Input: part model. Units: mm. Frame: model coordinates. A direction names the side the tool comes from. Coordinates: 2 decimals unless noted, no trailing zeros. Loops run counter-clockwise (first coordinate to the right, second up) from the corner with the lowest first, then second, coordinate; pieces in that order, holes last. Notation, with made-up numbers: (-28.5, -16.5) - (15.5, -16.5) arc R25 ccw to (15.5, 2.5) - close; hole circle Ø1 at (20.25, -14). An arc over 180 degrees is marked (long way). Use a Markdown table: item, result. Add a question column.
1. Section query C-C on x = 6. Return the cut outline in (y, z), then the cut area to 3 significant figures.
2. Section query A-A on y = 6. Return the cut outline in (x, z), then the cut area to 3 significant figures.
3. Access query for faces 1 (the face through (8.183, 20, 62)), 2 (the face through (15.183, 20, 62)), 3 (the face through (-23, 2, 52.899)), 4 (the face through (12, 20, -14.605)). Directions: +Z, -Z, +X, -X, +Y, -Y. A direction counts if a zero-diameter tool reaches every point of the face in a straight line with its end or side. Return the directions, or none.
4. Section query D-D on x = -46. Return the cut outline in (y, z).
5. Section query B-B on z = 23. State how many separate pieces and enclosed holes the cut face has, then the cut area to 3 significant figures.
6. Draft query along Z for faces 5 (the face through (17, 2, -7.101)), 6 (the face through (9, 12, 65.399)), 7 (the face through (4.383, 2, 23)), 8 (the face through (-47.817, 20, 23)). Return one class per face: released by +Z, released by -Z, zero draft, split by the parting line, or undercut.
7. Ray query, L1, parallel to Y at x = -18, z = 37.5; L2, parallel to X at y = 29, z = 62; L3, parallel to X at y = 30, z = 59. Return the intervals inside material, ascending. Write a range as [from, to].
8. Contact query for flat-ended pins moving along their axis: P1, Ø10, axis at x = 39, z = 14, coming from the +Y side; P2, Ø0.9, axis at y = 24.5, z = 61.5, coming from the +X side; P3, Ø2.5, axis at y = 13, z = 62, coming from the -X side. Output: stop coordinate, or through.
```python
from build123d import *

# Parameters (mm, degrees)
SKETCH3_W           = 105
SKETCH3_H           = 85
BOSS_EXTRUDE3_DEPTH = 3
SKETCH5_W           = 7
SKETCH5_H           = 7
SKETCH5_W_2         = 3
SKETCH5_H_2         = 3
BOSS_EXTRUDE4_DEPTH = 35
SKETCH9_W           = 2.998895248
SKETCH9_H           = 2.995380601
BOSS_EXTRUDE5_DEPTH = 35
SKETCH11_W          = 7
SKETCH11_H          = 7
SKETCH11_W_2        = 3
SKETCH11_H_2        = 3
BOSS_EXTRUDE6_DEPTH = 35
CUT_EXTRUDE1_DEPTH  = 6
SKETCH14_W          = 5
SKETCH14_H          = 60
CUT_EXTRUDE3_DEPTH  = 33
SKETCH17_W          = 5
SKETCH17_H          = 60
CUT_EXTRUDE4_DEPTH  = 15


with BuildPart() as part:
    # Sketch3 → Boss-Extrude3 (new body)
    with BuildSketch(Plane(origin=(0, 0, 0), x_dir=(1, 0, 0), z_dir=(0, 1, 0))):
        with Locations((-2.316884661, -22.898810939)):
            Rectangle(SKETCH3_W, SKETCH3_H)
    extrude(amount=BOSS_EXTRUDE3_DEPTH)

    # Sketch5 → Boss-Extrude4 (add)
    with BuildSketch(Plane(origin=(0, 3, 0), x_dir=(1, 0, 0), z_dir=(0, 1, 0))):
        with Locations((11.683115339, -61.898810939)):
            Rectangle(SKETCH5_W, SKETCH5_H)
        with Locations((11.683115339, -61.898810939)):
            Rectangle(SKETCH5_W_2, SKETCH5_H_2, mode=Mode.SUBTRACT)
    extrude(amount=BOSS_EXTRUDE4_DEPTH)

    # Sketch9 → Boss-Extrude5 (add)
    with BuildSketch(Plane(origin=(0, 3, 0), x_dir=(1, 0, 0), z_dir=(0, 1, 0))):
        Polygon((15.183115339, 12.601189061), (15.183115339, 19.601189061), (8.183115339, 19.601189061), (8.183115339, 17.600348451), (8.183115339, 12.601189061), align=None)
        with Locations((11.687877227, 16.102658151)):
            Rectangle(SKETCH9_W, SKETCH9_H, mode=Mode.SUBTRACT)
    extrude(amount=BOSS_EXTRUDE5_DEPTH)

    # Sketch11 → Boss-Extrude6 (add)
    with BuildSketch(Plane(origin=(0, 3, 0), x_dir=(1, 0, 0), z_dir=(0, 1, 0))):
        with Locations((-51.316884661, -22.898810939)):
            Rectangle(SKETCH11_W, SKETCH11_H)
        with Locations((-51.316884661, -22.898810939)):
            Rectangle(SKETCH11_W_2, SKETCH11_H_2, mode=Mode.SUBTRACT)
    extrude(amount=BOSS_EXTRUDE6_DEPTH)

    # Sketch12 → Cut-Extrude1 (cut)
    with BuildSketch(Plane(origin=(0, 3, 0), x_dir=(1, 0, 0), z_dir=(0, 1, 0))):
        Polygon((29.683115339, -52.898810939), (29.683115339, -48.898810939), (29.683115339, 3.101189061), (29.683115339, 7.101189061), (24.683115339, 7.101189061), (24.683115339, -52.898810939), align=None)
    extrude(amount=-CUT_EXTRUDE1_DEPTH, mode=Mode.SUBTRACT)

    # Sketch14 → Cut-Extrude3 (cut)
    with BuildSketch(Plane(origin=(0, 3, 0), x_dir=(1, 0, 0), z_dir=(0, 1, 0))):
        with Locations((17.183115339, -22.898810939)):
            Rectangle(SKETCH14_W, SKETCH14_H)
        with Locations((-2.816884661, -22.898810939)):
            Rectangle(SKETCH14_W, SKETCH14_H)
        with Locations((-22.816884661, -22.898810939)):
            Rectangle(SKETCH14_W, SKETCH14_H)
        with Locations((-12.816884661, -22.898810939)):
            Rectangle(SKETCH14_W, SKETCH14_H)
    extrude(amount=-CUT_EXTRUDE3_DEPTH, mode=Mode.SUBTRACT)

    # Sketch17 → Cut-Extrude4 (cut)
    with BuildSketch(Plane(origin=(0, 3, 0), x_dir=(1, 0, 0), z_dir=(0, 1, 0))):
        with Locations((6.882849783, -22.898810939)):
            Rectangle(SKETCH17_W, SKETCH17_H)
    extrude(amount=-CUT_EXTRUDE4_DEPTH, mode=Mode.SUBTRACT)


solid = part.part
```
Resolved:
| question | item | result |
|---|---|---|
| 1 | outline | (0, -19.6) - (3, -19.6) - (3, -7.1) - (0, -7.1) - close; (0, 52.9) - (3, 52.9) - (3, 65.4) - (0, 65.4) - close |
| 1 | area | 75.0 mm² |
| 2 | outline | (-54.82, 19.4) - (-47.82, 19.4) - (-47.82, 26.4) - (-54.82, 26.4) - close; (8.18, -19.6) - (15.18, -19.6) - (15.18, -12.6) - (8.18, -12.6) - close; (8.18, 58.4) - (15.18, 58.4) - (15.18, 65.4) - (8.18, 65.4) - close; hole (-52.82, 21.4) - (-49.82, 21.4) - (-49.82, 24.4) - (-52.82, 24.4) - close; hole (10.18, 60.4) - (13.18, 60.4) - (13.18, 63.4) - (10.18, 63.4) - close; hole (10.19, -17.6) - (13.19, -17.6) - (13.19, -14.6) - (10.19, -14.6) - close |
| 2 | area | 120 mm² |
| 3 | face 1 | +Z, -Z, -X, +Y |
| 3 | face 2 | +Z, -Z, +X, +Y |
| 3 | face 3 | +Y, -Y |
| 3 | face 4 | +Y |
| 4 | outline | (0, -19.6) - (3, -19.6) - (3, 65.4) - (0, 65.4) - close |
| 5 | separate pieces | 7 |
| 5 | enclosed holes | 0 |
| 5 | area | 365 mm² |
| 6 | face 5 | undercut |
| 6 | face 6 | released by +Z |
| 6 | face 7 | undercut |
| 6 | face 8 | zero draft |
| 7 | L1 | [0, 3] |
| 7 | L2 | [8.18, 10.18], [13.18, 15.18] |
| 7 | L3 | [8.18, 15.18] |
| 8 | P1 | y = 3 |
| 8 | P2 | x = 15.18 |
| 8 | P3 | x = 8.18 |
